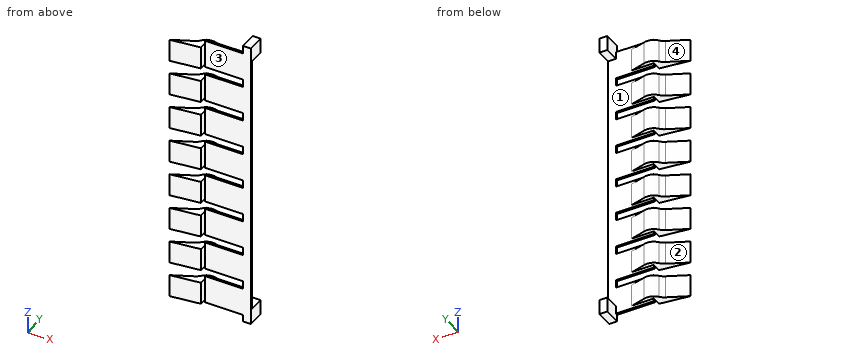
```python
from build123d import *

# Parameters (mm, degrees)
EXTRUDE1_DEPTH       = 11.25
SKETCH3_W            = 22.5
SKETCH3_H            = 5.033767183
EXTRUDE2_DEPTH       = 10
EXTRUDE3_DEPTH       = 14
SKETCH5_W            = 10
SKETCH5_H            = 2
EXTRUDE4_DEPTH       = 167.995
LPATTERN1_OUTLINE_W  = 2
LPATTERN1_OUTLINE_H  = 28
LPATTERN1_DEPTH      = 36
EXTRUDE6_DEPTH       = 175.64601587
EXTRUDE6_DEPTH_BACK  = 175.64601587
SKETCH7_W            = 3
SKETCH7_H            = 2
EXTRUDE7_DEPTH       = 36
LPATTERN2_COUNT      = 4
LPATTERN2_PITCH      = 36
LPATTERN2_COUNT_DIR2 = 5
LPATTERN2_PITCH_DIR2 = 36
SKETCH8_W            = 2
SKETCH8_H            = 6.995
SKETCH8_H_2          = 8
EXTRUDE8_DEPTH       = 175.64601587
EXTRUDE9_DEPTH       = 175.64601587
SKETCH10_W           = 7.252078552
SKETCH10_H           = 8.610092753
EXTRUDE10_DEPTH      = 290.080499228
SKETCH11_W           = 8
SKETCH11_H           = 15
EXTRUDE11_DEPTH      = 15


# Read off the part's stored shape, not the designer's step: LPattern1
with BuildPart() as part:
    # Sketch1 → Extrude1 (new, symmetric)
    with BuildSketch(Plane.XY):
        with BuildLine():
            Line((22.243678564, 3.6), (7.8688831, 7.451714836))
            ThreePointArc((7.8688831, 7.451714836), (0.766318838, 7.515222423), (-5.127958891, 3.551897764))
            ThreePointArc((-5.127958891, 3.551897764), (-7.125613619, 1.593106665), (-9.522547255, 0.150124985))
            ThreePointArc((-9.522547255, 0.150124985), (-9.563578628, 0.131412483), (-9.604503865, 0.11246898))
            Line((-9.604503865, 0.11246898), (-29.497211353, -9.163652863))
            Line((-29.497211353, -9.163652863), (4.045876789, -5.033767183))
            Line((4.045876789, -5.033767183), (4.045876789, 0))
            Line((4.045876789, 0), (0, 0))
            Line((0, 0), (0, 3.6))
            Line((0, 3.6), (22.243678564, 3.6))
        make_face()
    extrude1 = extrude(amount=EXTRUDE1_DEPTH, both=True)

    # Sketch3 → Extrude2 (cut)
    with BuildSketch(Plane(origin=(4.045876789, 0, 0), x_dir=(0, 0, -1), z_dir=(1, 0, 0))):
        with Locations((0, -2.516883592)):
            Rectangle(SKETCH3_W, SKETCH3_H)
    extrude(amount=-EXTRUDE2_DEPTH, mode=Mode.SUBTRACT)

    # Sketch4 → Extrude3 (add, symmetric)
    with BuildSketch(Plane.XY):
        Polygon((0, 1.6), (0, 3.6), (22.243678564, 3.6), (36, 3.6), (36, 1.6), align=None)
    extrude(amount=EXTRUDE3_DEPTH, both=True)

    # Sketch5 → Extrude4 (add, symmetric)
    with BuildSketch(Plane.XY):
        with Locations((41, 2.6)):
            Rectangle(SKETCH5_W, SKETCH5_H)
    extrude(amount=EXTRUDE4_DEPTH, both=True)

    # LPattern1 outline → LPattern1 (add)
    with BuildSketch(Plane.YZ):
        with Locations((2.6, -144)):
            Rectangle(LPATTERN1_OUTLINE_W, LPATTERN1_OUTLINE_H)
        with Locations((2.6, -108)):
            Rectangle(LPATTERN1_OUTLINE_W, LPATTERN1_OUTLINE_H)
        with Locations((2.6, -72)):
            Rectangle(LPATTERN1_OUTLINE_W, LPATTERN1_OUTLINE_H)
        with Locations((2.6, -36)):
            Rectangle(LPATTERN1_OUTLINE_W, LPATTERN1_OUTLINE_H)
        with Locations((2.6, 36)):
            Rectangle(LPATTERN1_OUTLINE_W, LPATTERN1_OUTLINE_H)
        with Locations((2.6, 72)):
            Rectangle(LPATTERN1_OUTLINE_W, LPATTERN1_OUTLINE_H)
        with Locations((2.6, 108)):
            Rectangle(LPATTERN1_OUTLINE_W, LPATTERN1_OUTLINE_H)
        with Locations((2.6, 144)):
            Rectangle(LPATTERN1_OUTLINE_W, LPATTERN1_OUTLINE_H)
    extrude(amount=LPATTERN1_DEPTH)

    # Sketch6 → Extrude6 (cut, two sides: drawn at the far end of the back side and taken through both)
    with BuildSketch(Plane(origin=(0, 3.6, 0), x_dir=(1, 0, 0), z_dir=(0, 1, 0)).offset(-EXTRUDE6_DEPTH_BACK)):
        Polygon((-630.637797583, -133), (0, -133), (46, -133), (676.637797583, -133), (676.637797583, -1394.275595165), (-630.637797583, -1394.275595165), align=None)
    extrude(amount=EXTRUDE6_DEPTH + EXTRUDE6_DEPTH_BACK, mode=Mode.SUBTRACT)

    # Sketch7 → Extrude7 (add)
    with BuildSketch(Plane.ZY.offset(-36)):
        with Locations((-166.495, 2.6)):
            Rectangle(SKETCH7_W, SKETCH7_H)
    extrude(amount=EXTRUDE7_DEPTH)

    # LPattern2: Extrude1 4 × 5
    with Locations(*[Vector(0, 0, 1) * (i * LPATTERN2_PITCH) + Vector(0, 0, -1) * (j * LPATTERN2_PITCH_DIR2) for i in range(LPATTERN2_COUNT) for j in range(LPATTERN2_COUNT_DIR2) if (i, j) != (0, 0)]):
        add(extrude1)

    # Sketch8 → Extrude8 (cut, through all)
    with BuildSketch(Plane(origin=(0, 3.6, 0), x_dir=(1, 0, 0), z_dir=(0, 1, 0))):
        with Locations((37, 161.4975)):
            Rectangle(SKETCH8_W, SKETCH8_H)
        with Locations((37, 126)):
            Rectangle(SKETCH8_W, SKETCH8_H_2)
        with Locations((37, 90)):
            Rectangle(SKETCH8_W, SKETCH8_H_2)
        with Locations((37, 54)):
            Rectangle(SKETCH8_W, SKETCH8_H_2)
        with Locations((37, 18)):
            Rectangle(SKETCH8_W, SKETCH8_H_2)
        with Locations((37, -18)):
            Rectangle(SKETCH8_W, SKETCH8_H_2)
        with Locations((37, -54)):
            Rectangle(SKETCH8_W, SKETCH8_H_2)
        with Locations((37, -90)):
            Rectangle(SKETCH8_W, SKETCH8_H_2)
        with Locations((37, -126)):
            Rectangle(SKETCH8_W, SKETCH8_H_2)
    extrude(amount=-EXTRUDE8_DEPTH, mode=Mode.SUBTRACT)

    # Sketch9 → Extrude9 (cut, through all)
    with BuildSketch(Plane(origin=(0, 3.6, 0), x_dir=(1, 0, 0), z_dir=(0, 1, 0))):
        Polygon((38, 164.995), (46, 164.995), (46, 167.995), (0, 167.995), (0, 164.995), align=None)
        Polygon((38, -130), (46, -130), (46, -133), (0, -133), (0, -130), align=None)
    extrude(amount=-EXTRUDE9_DEPTH, mode=Mode.SUBTRACT)

    # Sketch10 → Extrude10 (cut, through all)
    with BuildSketch(Plane(origin=(0, 0, -155.25), x_dir=(-1, 0, 0), z_dir=(0, 0, -1))):
        with Locations((-3.626039276, -2.705046377)):
            Rectangle(SKETCH10_W, SKETCH10_H)
    extrude(amount=-EXTRUDE10_DEPTH, mode=Mode.SUBTRACT)

    # Sketch11 → Extrude11 (add)
    with BuildSketch(Plane(origin=(0, 3.6, 0), x_dir=(1, 0, 0), z_dir=(0, 1, 0))):
        with Locations((42, 157.495)):
            Rectangle(SKETCH11_W, SKETCH11_H)
        with Locations((42, -122.5)):
            Rectangle(SKETCH11_W, SKETCH11_H)
    extrude(amount=EXTRUDE11_DEPTH)


solid = part.part
```
For this review, take the finished solid that the model builds, in its own axes (mm). Face numbers are marked on the shaded views. A direction names the side the tool comes from. Round coordinates to 2 decimals unless told otherwise and drop trailing zeros. Write each loop counter-clockwise with the first axis right and the second up, starting at its lowest first coordinate (ties: lowest second). Pieces come first, ordered by that corner, then holes. Notation, with made-up numbers: (1.25, 37) -> (37.25, 37) arc R10 ccw to (37.25, 50) -> close; hole circle Ø9 at (3.5, 6). An arc over 180 degrees is marked (long way). Use one line per item in the form item = value.
Q1. Consider section C-C (z = 100.5). State the section outline as (x, y) points, then the cut area to 3 significant figures.
Resolved:
outline = (-29.5, -9.16) -> (0, -5.53) -> (0, 1.6) -> (46, 1.6) -> (46, 3.6) -> (22.24, 3.6) -> (7.87, 7.45) arc R12 ccw to (-5.13, 3.55) arc R12 cw to (-9.52, 0.15) arc R8 ccw to (-9.6, 0.11) -> close
area = 316 mm²
Q2. Clearance check with flat-ended pins moving along their axes: pin 1 Ø0.6 at (x, y) = (11.5, 3) entering from +Z; pin 2 Ø2 at (y, z) = (3, 95.5) entering from -X; pin 3 Ø2 at (x, z) = (-5, 75) entering from -Y; pin 4 Ø1.5 at (y, z) = (4, 12) entering from +X. State where each tip first meets the part, or that it passes through.
Resolved:
pin_1 = 122
pin_2 = 0
pin_3 = -6.27
pin_4 = 46
Q3. Consider section A-A (y = 14.25). State the section outline as (x, z) points (3 decimals).
Resolved:
outline = (38, -164.995) -> (46, -164.995) -> (46, -149.995) -> (38, -149.995) -> close; (38, 115) -> (46, 115) -> (46, 130) -> (38, 130) -> close
Q4. Machinability: for the marked faces 3 and 4, which of the approach directions +Z, -Z, +X, -X, +Y, -Y give a long, thin tool a straight path to every point of the face, cutting with its end or side? Answer none if there is none.
Resolved:
face_3 = +Z, -Z, +X, -Y
face_4 = +Z, -Z, -X, +Y
Q5. The part is to be moulded in two halves that separate along Z. For the marked faces 1 and 2, say which applies: released by +Z, released by -Z, zero draft, split by the parting line, or undercut.
Resolved:
face_1 = undercut
face_2 = zero draft
Q6. Consider section B-B (x = 34). State how many separate pieces and enclosed holes the cut face has, then the cut area to 3 significant figures.
Resolved:
separate_pieces = 8
enclosed_holes = 0
area = 448 mm²
Q7. To check wall thickness, follow probe 1 along Y at (x, z) = (23, -4.5); probe 2 along Y at (x, z) = (6, -142); probe 3 along X at (y, z) = (3, -131). State the ranges of each line that lie inside material, in increasing order. Write a range as from..to.
Resolved:
probe_1 = 1.6..3.6
probe_2 = 1.6..7.89
probe_3 = 0..46
